For this review, take the finished solid that the model builds, in its own axes (mm). Give positions to 0.01 mm unless a question says otherwise; leave off trailing zeros. Loops run counter-clockwise (first coordinate to the right, second up) from the corner with the lowest first, then second, coordinate; pieces in that order, holes last.
Autodesk Inventor part; units mm, degrees
ref_plane "Work Plane1" through (0, 0, 1.5) normal (0, 0, 1) x (1, 0, 0)
ref_plane "YZ Plane" through (0, 0, 0) normal (1, 0, 0) x (0, 1, 0)
ref_plane "XZ Plane" through (0, 0, 0) normal (0, 1, 0) x (-1, 0, 0)
sketch "Sketch1" plane through (0, 0, 0) normal (0, 0, 1) x (1, 0, 0)
  line L0 (-13.9785, 19.8477) -> (4.0215, 19.8477)
  line L1 (4.0215, -20.1523) -> (-13.9785, -20.1523)
  line L2 (-13.9785, -20.1523) -> (-13.9785, 19.8477)
  line L3 (6.0215, -22.1523) -> (6.0215, -38.1523)
  line L4 (6.0215, 21.8477) -> (6.0215, 32.8477)
  circle A0 centre (-3.9785, -10.9023) radius 2.5
  line L5 (6.0215, 19.8477) -> (6.0215, 34.8477)
  line L6 (6.0215, -20.1523) -> (6.0215, -40.1523)
  line L7 (4.0215, -40.1523) -> (-1.9785, -40.1523)
  line L8 (-3.9785, -80.9023) -> (-3.9785, -95.9023)
  line L9 (-3.9785, -98.9023) -> (-3.9785, -42.1523)
  line L10 (-23.9785, 32.8477) -> (-23.9785, -75.9023)
  line L11 (6.0215, 19.8477) -> (6.0215, 34.8477)
  circle A1 centre (-8.9785, -24.1523) radius 1.5
  circle A2 centre (1.0215, -24.1523) radius 1.5
  circle A3 centre (-8.9785, 23.8477) radius 1.5
  circle A4 centre (1.0215, 23.8477) radius 1.5
  line L12 (-5.9785, -100.9023) -> (-16.9785, -100.9023)
  line L13 (6.0215, 19.8477) -> (6.0215, 21.4291)
  line L14 (6.0215, 19.8477) -> (6.0215, 34.8477)
  line L15 (4.0215, 34.8477) -> (-21.9785, 34.8477)
  line L16 (-18.9785, -98.9023) -> (-18.9785, -84.5626)
  line L17 (-18.9785, -80.9023) -> (-18.9785, -80.9023)
  arc A5 (-18.9785, -98.9023) -> (-16.9785, -100.9023) centre (-16.9785, -98.9023) ccw
  arc A6 (-5.9785, -100.9023) -> (-3.9785, -98.9023) centre (-5.9785, -98.9023) ccw
  arc A7 (-1.9785, -40.1523) -> (-3.9785, -42.1523) centre (-1.9785, -42.1523) ccw
  arc A8 (4.0215, -40.1523) -> (6.0215, -38.1523) centre (4.0215, -38.1523) ccw
  arc A9 (6.0215, -22.1523) -> (4.0215, -20.1523) centre (4.0215, -22.1523) ccw
  arc A10 (4.0215, 19.8477) -> (6.0215, 21.8477) centre (4.0215, 21.8477) ccw
  arc A11 (6.0215, 32.8477) -> (4.0215, 34.8477) centre (4.0215, 32.8477) ccw
  arc A12 (-21.9785, 34.8477) -> (-23.9785, 32.8477) centre (-21.9785, 32.8477) ccw
  arc A13 (-23.9785, -75.9023) -> (-21.4785, -80.2325) centre (-18.9785, -75.9023) ccw
  arc A14 (-18.9785, -84.5626) -> (-21.4785, -80.2325) centre (-23.9785, -84.5626) ccw
  circle A15 centre (-13.9785, -50.1523) radius 1.5
  circle A16 centre (-11.4785, -84.5626) radius 1.5
  point P0 (0, 0)
  point P1 (0, 0)
  point P2 (0, 0)
  point P3 (-23.9785, 34.8477)
  point P4 (-3.9785, -100.9023)
  point P5 (-18.9785, -100.9023)
  dimension "d0" = 5
  dimension "d1" = 20
  dimension "d2" = 3
  dimension "d3" = 5
  dimension "d4" = 4
  dimension "d5" = 3
  dimension "d6" = 10
  dimension "d7" = 3
  dimension "d8" = 3
  dimension "d9" = 10
  dimension "d10" = 5
  dimension "d11" = 4
  dimension "d14" = 15
  dimension "d15" = 135.75
  dimension "d18" = 10
  dimension "d19" = 15
  dimension "d21" = 30
  dimension "d22" = 2
  dimension "d23" = 5
  dimension "d26" = 3
  dimension "d27" = 3
  dimension "d29" = 30
  dimension "d62" = 48
  dimension "d63" = 48
extrude "Extrusion2" add sketch "Sketch1" along normal blind 1.5 contours L2 L1 A9 L3 A8 L7 A7 L9 L8 A6 L12 A5 L16 A14 A13 L10 A12 L15 A11 L4 A10 L0 | A1 | A2 | A3 | A4 | A15 | A16
ref_plane "Work Plane1" through (0, 0, 1.5) normal (0, 0, 1) x (1, 0, 0)
sketch "Sketch4" plane through (0, 0, 1.5) normal (0, 0, 1) x (1, 0, 0)
  line L0 (-13.9785, 19.8477) -> (4.0215, 19.8477)
  line L1 (4.0215, -20.1523) -> (-13.9785, -20.1523)
  line L2 (-13.9785, -20.1523) -> (-13.9785, 19.8477)
  line L3 (6.0215, -22.1523) -> (6.0215, -38.1523)
  line L4 (6.0215, 21.8477) -> (6.0215, 32.8477)
  circle A0 centre (-3.9785, -10.9023) radius 2.5
  line L5 (6.0215, 19.8477) -> (6.0215, 34.8477)
  line L6 (6.0215, -20.1523) -> (6.0215, -40.1523)
  line L7 (4.0215, -40.1523) -> (-1.9785, -40.1523)
  line L8 (-3.9785, -80.9023) -> (-3.9785, -95.9023)
  line L9 (-3.9785, -98.9023) -> (-3.9785, -42.1523)
  line L10 (-23.9785, 32.8477) -> (-23.9785, -75.9023)
  line L11 (6.0215, 19.8477) -> (6.0215, 34.8477)
  circle A1 centre (-8.9785, -24.1523) radius 1.5
  circle A2 centre (1.0215, -24.1523) radius 1.5
  circle A3 centre (-8.9785, 23.8477) radius 1.5
  circle A4 centre (1.0215, 23.8477) radius 1.5
  line L12 (-5.9785, -100.9023) -> (-16.9785, -100.9023)
  line L13 (6.0215, 19.8477) -> (6.0215, 21.4291)
  line L14 (6.0215, 19.8477) -> (6.0215, 34.8477)
  line L15 (4.0215, 34.8477) -> (-21.9785, 34.8477)
  line L16 (-18.9785, -98.9023) -> (-18.9785, -84.5626)
  line L17 (-18.9785, -80.9023) -> (-18.9785, -80.9023)
  arc A5 (-18.9785, -98.9023) -> (-16.9785, -100.9023) centre (-16.9785, -98.9023) ccw
  arc A6 (-5.9785, -100.9023) -> (-3.9785, -98.9023) centre (-5.9785, -98.9023) ccw
  arc A7 (-1.9785, -40.1523) -> (-3.9785, -42.1523) centre (-1.9785, -42.1523) ccw
  arc A8 (4.0215, -40.1523) -> (6.0215, -38.1523) centre (4.0215, -38.1523) ccw
  arc A9 (6.0215, -22.1523) -> (4.0215, -20.1523) centre (4.0215, -22.1523) ccw
  arc A10 (4.0215, 19.8477) -> (6.0215, 21.8477) centre (4.0215, 21.8477) ccw
  arc A11 (6.0215, 32.8477) -> (4.0215, 34.8477) centre (4.0215, 32.8477) ccw
  arc A12 (-21.9785, 34.8477) -> (-23.9785, 32.8477) centre (-21.9785, 32.8477) ccw
  arc A13 (-23.9785, -75.9023) -> (-21.4785, -80.2325) centre (-18.9785, -75.9023) ccw
  arc A14 (-18.9785, -84.5626) -> (-21.4785, -80.2325) centre (-23.9785, -84.5626) ccw
  circle A15 centre (-13.9785, -50.1523) radius 1.5
  circle A16 centre (-11.4785, -84.5626) radius 1.5
  point P0 (0, 0)
  point P1 (0, 0)
  point P2 (0, 0)
  point P3 (0, 0)
  point P4 (-23.9785, 34.8477)
  point P5 (-3.9785, -100.9023)
  point P6 (-18.9785, -100.9023)
  dimension "d33" = 5
  dimension "d34" = 20
  dimension "d35" = 3
  dimension "d36" = 5
  dimension "d37" = 4
  dimension "d38" = 3
  dimension "d39" = 10
  dimension "d40" = 3
  dimension "d41" = 3
  dimension "d42" = 10
  dimension "d43" = 5
  dimension "d44" = 4
  dimension "d45" = 15
  dimension "d46" = 135.75
  dimension "d47" = 10
  dimension "d48" = 15
  dimension "d49" = 30
  dimension "d50" = 2
  dimension "d51" = 5
  dimension "d52" = 3
  dimension "d53" = 3
  dimension "d54" = 30
hole "Hole1" at (-8.9785, 23.8477, 1.5) at (1.0215, 23.8477, 1.5) at (-8.9785, -24.1523, 1.5) at (1.0215, -24.1523, 1.5) at (-13.9785, -50.1523, 1.5) at (-11.4785, -84.5626, 1.5) direction (0, 0, -1) diameter 3 end through all
properties part number "riset tibia alumunium 1"
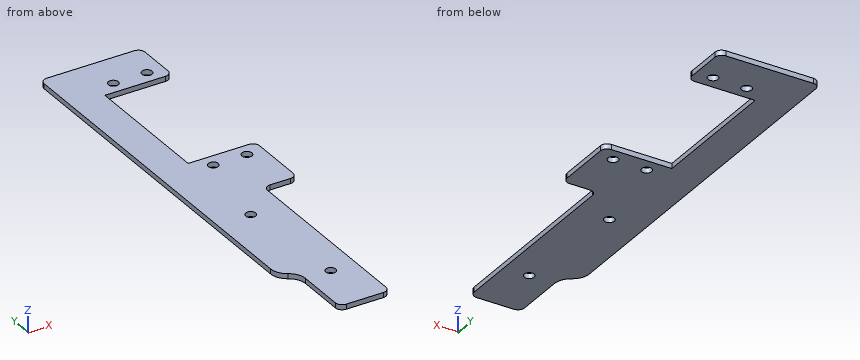
Q1. For probe 1 along Y at (x, z) = (1, 0.35); probe 2 along Y at (x, z) = (-9, 1.05); probe 3 along Y at (x, z) = (2.75, 0.65), list the stretches that pass through material, from the lowest coordinate up.
Answers:
probe 1: y = -40.15 to -25.65, -22.65 to -20.15, 19.85 to 22.35, 25.35 to 34.85
probe 2: y = -100.9 to -25.65, -22.65 to -20.15, 19.85 to 22.35, 25.35 to 34.85
probe 3: y = -40.15 to -20.15, 19.85 to 34.85
Q2. Consider section B-B on z = 1. Give the boundary of the cut face in (x, y).
Answers:
outline: (-23.98, -75.9) arc R5 ccw to (-21.48, -80.23) arc R5 cw to (-18.98, -84.56) - (-18.98, -98.9) arc R2 ccw to (-16.98, -100.9) - (-5.98, -100.9) arc R2 ccw to (-3.98, -98.9) - (-3.98, -42.15) arc R2 cw to (-1.98, -40.15) - (4.02, -40.15) arc R2 ccw to (6.02, -38.15) - (6.02, -22.15) arc R2 ccw to (4.02, -20.15) - (-13.98, -20.15) - (-13.98, 19.85) - (4.02, 19.85) arc R2 ccw to (6.02, 21.85) - (6.02, 32.85) arc R2 ccw to (4.02, 34.85) - (-21.98, 34.85) arc R2 ccw to (-23.98, 32.85) - close; hole circle Ø3 at (-13.98, -50.15); hole circle Ø3 at (-11.48, -84.56); hole circle Ø3 at (-8.98, -24.15); hole circle Ø3 at (-8.98, 23.85); hole circle Ø3 at (1.02, -24.15); hole circle Ø3 at (1.02, 23.85)
Q3. For pin 1 Ø0.8 at (x, z) = (2, 1) entering from -Y; pin 2 Ø0.8 at (y, z) = (-10, 1) entering from +X; pin 3 Ø0.8 at (y, z) = (-90, 0.5) entering from -X, all flat-tipped, find the tip position at first contact; note any pin that passes through.
Answers:
pin 1: stops at y = -40.15
pin 2: stops at x = -13.98
pin 3: stops at x = -18.98
Q4. Consider section A-A on y = 12. Give the boundary of the cut face in (x, z).
Answers:
outline: (-23.98, 0) - (-13.98, 0) - (-13.98, 1.5) - (-23.98, 1.5) - close
